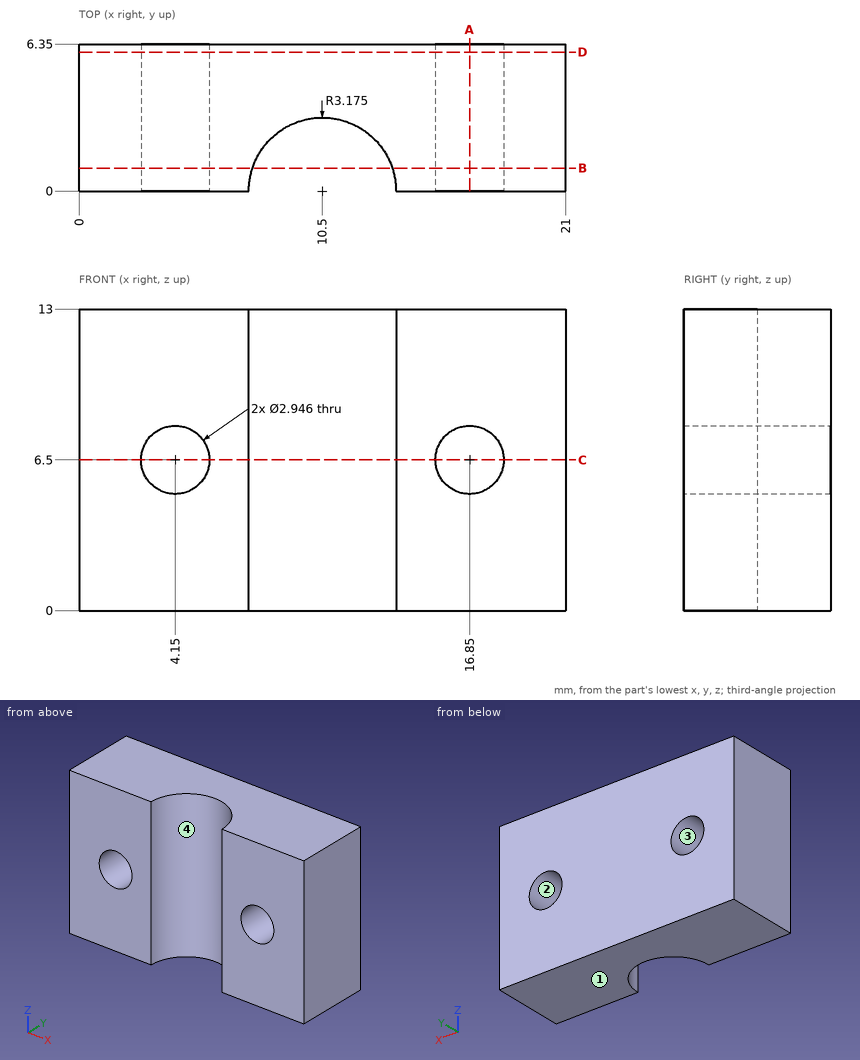
Could you check a few things on this drawing? It's one solid part, dimensions in mm from its lowest x, y, z. Round coordinates to 2 decimals unless told otherwise and drop trailing zeros. Loops run counter-clockwise (first coordinate to the right, second up) from the corner with the lowest first, then second, coordinate; pieces in that order, holes last.
Q1. Please list where these lines run through material, in increasing order: L1, parallel to X at y = 4.5, z = 6.5; L2, parallel to X at y = 2.25, z = 6.5 (1 decimal); L3, parallel to Z at x = 16.25, y = 4.5 (1 decimal).
Q2. Thinking about a two-plate mould opening in Z: for the marked faces 1, 2, 3 and 4, which applies, pulls with the +Z half, pulls with the -Z half, needs draft (parallel to the pull), parting line crosses it, or undercut?
Q3. I want a section at D-D (y = 6). Write out the boundary of the cut face in (x, z), and give its area (3 significant figures).
Q4. I want a section at C-C (z = 6.5). Give the number of separate pieces and of enclosed holes in the cut face.
Q5. I want a section at A-A (x = 16.85). Write out the boundary of the cut face in (y, z).
Q6. I want a section at B-B (y = 1). Write out the boundary of the cut face in (x, z).
Answer below:
1. L1: x = 0 to 2.68, 5.62 to 15.38, 18.32 to 21
1. L2: x = 0 to 2.7, 5.6 to 8.3, 12.7 to 15.4, 18.3 to 21
1. L3: z = 0 to 5.2, 7.8 to 13
2. face 1: pulls with the -Z half
2. face 2: undercut
2. face 3: undercut
2. face 4: needs draft
3. outline: (0, 0) - (21, 0) - (21, 13) - (0, 13) - close; hole circle Ø2.95 at (4.15, 6.5); hole circle Ø2.95 at (16.85, 6.5)
3. area: 259 mm2
4. separate pieces: 3
4. enclosed holes: 0
5. outline: (0, 0) - (6.35, 0) - (6.35, 5.03) - (0, 5.03) - close; (0, 7.97) - (6.35, 7.97) - (6.35, 13) - (0, 13) - close
6. outline: (0, 0) - (7.49, 0) - (7.49, 13) - (0, 13) - close; (13.51, 0) - (21, 0) - (21, 13) - (13.51, 13) - close; hole circle Ø2.95 at (4.15, 6.5); hole circle Ø2.95 at (16.85, 6.5)
